For this review, take the finished solid that the model builds, in its own axes (mm). Give positions to 0.01 mm unless a question says otherwise; leave off trailing zeros. Loops run counter-clockwise (first coordinate to the right, second up) from the corner with the lowest first, then second, coordinate; pieces in that order, holes last. Notation, with made-up numbers: (30.25, 75.5) -> (87.25, 75.5) arc R18 ccw to (87.25, 95.5) -> close; hole circle Ø2 at (83.25, 81.25). An arc over 180 degrees is marked (long way). One line per question, with ' | ' between items. Start each with the question number.
(1) Consider section C-C (z = 14). Write out the cut boundary in (x, y).
(2) Consider section B-B (z = 2). Write out the cut boundary in (x, y).
(3) Wall thickness on probe 1 along Z at (x, y) = (59.5, 0.5); probe 2 along X at (y, z) = (2.85, 2.5); probe 3 along Z at (x, y) = (-61.5, 1.9): over which ranges is each line inside the solid? List them lowest first.
(4) Consider section D-D (y = 1.05). Give the number of separate pieces and of enclosed holes in the cut face, and give its area (3 significant figures).
(5) Consider section A-A (x = 59.5). Write out the cut boundary in (y, z), and give its area (3 significant figures).
(6) Insertion check: P1, Ø3.5, axis at x = 6.22, z = -8.15, coming from the -Y side; P2, Ø0.9, axis at y = 1, z = -27, coming from the +X side; P3, Ø0.9, axis at y = 2, z = -31.5, coming from the -X side. Each pin has a flat end and moves straight along its axis. Give the tip position at first contact, or say it passes through.
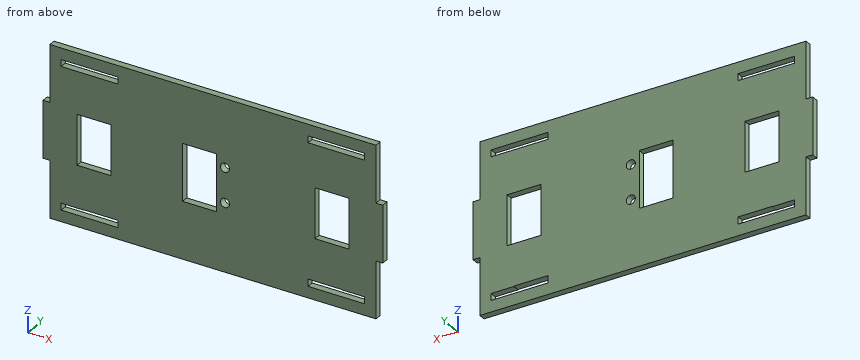
Autodesk Inventor part; units mm, degrees
ref_plane "YZ Plane" through (0, 0, 0) normal (1, 0, 0) x (0, 1, 0)
ref_plane "XZ Plane" through (0, 0, 0) normal (0, 1, 0) x (-1, 0, 0)
ref_plane "XY Plane" through (0, 0, 0) normal (0, 0, 1) x (1, 0, 0)
sketch "Sketch1" plane through (0, 0, 0) normal (0, 1, 0) x (-1, 0, 0)
  line L0 (71.1097, -38.0648) -> (71.1097, -13.0648)
  line L1 (71.1097, -13.0648) -> (74.1097, -13.0648)
  line L2 (74.1097, -13.0648) -> (74.1097, 11.9352)
  line L3 (74.1097, 11.9352) -> (71.1097, 11.9352)
  line L4 (71.1097, 11.9352) -> (71.1097, 36.9352)
  line L5 (-72.8903, -38.0648) -> (-72.8903, -13.0648)
  line L6 (-72.8903, 36.9352) -> (-72.8903, 11.9352)
  line L7 (-72.8903, -13.0648) -> (-75.8903, -13.0648)
  line L8 (-75.8903, -13.0648) -> (-75.8903, 11.9352)
  line L9 (-75.8903, 11.9352) -> (-72.8903, 11.9352)
  line L10 (71.1097, -38.0648) -> (-72.8903, -38.0648)
  line L11 (71.1097, 36.9352) -> (-72.8903, 36.9352)
  point P0 (0, 0)
extrude "Extrusion1" add sketch "Sketch1" along normal blind 3
sketch "Sketch2" plane through (0, 3, 0) normal (0, 1, 0) x (1, 0, 0)
  line L0 (-71.1097, -36.9352) -> (72.8903, -36.9352)
  line L1 (-66.1097, -31.9352) -> (-56.1097, -31.9352)
  line L2 (-56.1097, -31.9352) -> (-56.1097, -28.9352)
  line L3 (-56.1097, -28.9352) -> (-66.1097, -28.9352)
  line L4 (-66.1097, -28.9352) -> (-66.1097, -31.9352)
  line L5 (72.8903, 38.0648) -> (-71.1097, 38.0648)
  line L6 (-56.1097, 30.0648) -> (-66.1097, 30.0648)
  line L7 (-66.1097, 30.0648) -> (-66.1097, 33.0648)
  line L8 (-66.1097, 33.0648) -> (-56.1097, 33.0648)
  line L9 (-56.1097, 33.0648) -> (-56.1097, 30.0648)
  line L10 (67.8903, 33.0648) -> (57.8903, 33.0648)
  line L11 (57.8903, 33.0648) -> (57.8903, 30.0648)
  line L12 (57.8903, 30.0648) -> (67.8903, 30.0648)
  line L13 (67.8903, 30.0648) -> (67.8903, 33.0648)
  line L14 (67.8903, -31.9352) -> (57.8903, -31.9352)
  line L15 (57.8903, -31.9352) -> (57.8903, -28.9352)
  line L16 (57.8903, -28.9352) -> (67.8903, -28.9352)
  line L17 (67.8903, -28.9352) -> (67.8903, -31.9352)
  point P0 (0, 0)
extrude "Extrusion2" cut sketch "Sketch2" against normal blind 30
sketch "Sketch3" plane through (0, 3, 0) normal (0, 1, 0) x (1, 0, 0)
  line L0 (72.8903, 38.0648) -> (-71.1097, 38.0648)
  line L1 (-71.1097, -36.9352) -> (72.8903, -36.9352)
  line L2 (-74.1097, 13.0648) -> (-74.1097, -11.9352)
  line L3 (75.8903, -11.9352) -> (75.8903, 13.0648)
  circle A0 centre (6.2215, -7.0252) radius 2
  circle A1 centre (6.2215, 8.1548) radius 2
  line L4 (2.4888, 13.0648) -> (-12.5112, 13.0648)
  line L5 (-12.5112, 13.0648) -> (-12.5112, -11.9352)
  line L6 (-12.5112, -11.9352) -> (2.4888, -11.9352)
  line L7 (2.4888, -11.9352) -> (2.4888, 13.0648)
  line L8 (-59.1097, -10.4352) -> (-44.1097, -10.4352)
  line L9 (-44.1097, -10.4352) -> (-44.1097, 11.5648)
  line L10 (-44.1097, 11.5648) -> (-59.1097, 11.5648)
  line L11 (-59.1097, 11.5648) -> (-59.1097, -10.4352)
  line L12 (60.8903, 11.5648) -> (45.8903, 11.5648)
  line L13 (45.8903, 11.5648) -> (45.8903, -10.4352)
  line L14 (45.8903, -10.4352) -> (60.8903, -10.4352)
  line L15 (60.8903, -10.4352) -> (60.8903, 11.5648)
  point P0 (0, 0)
  dimension "d56" = 15
  dimension "d57" = 22
  dimension "d59" = 25
  dimension "d60" = 15
  dimension "d61" = 4
  dimension "d62" = 4
  dimension "d63" = 15
  dimension "d64" = 22
extrude "Extrusion3" cut sketch "Sketch3" against normal blind 10
sketch "Sketch4" plane through (0, 3, 0) normal (0, 1, 0) x (1, 0, 0)
  line L0 (-56.1097, 33.0648) -> (-41.1097, 33.0648)
  line L1 (-41.1097, 33.0648) -> (-41.1097, 29.924)
  line L2 (-41.1097, 29.924) -> (-56.1097, 29.924)
  line L3 (-56.1097, 29.924) -> (-56.1097, 33.0648)
  line L4 (57.8903, 30.0648) -> (57.8903, 33.0648)
  line L5 (57.8903, 33.0648) -> (42.8903, 33.0648)
  line L6 (42.8903, 33.0648) -> (42.8903, 29.924)
  line L7 (42.8903, 29.924) -> (57.8903, 29.924)
  line L8 (57.8903, 29.924) -> (57.8903, 33.0648)
  line L9 (-56.1097, -31.9352) -> (-41.1097, -31.9352)
  line L10 (-41.1097, -31.9352) -> (-41.1097, -28.9352)
  line L11 (-41.1097, -28.9352) -> (-56.1097, -28.9352)
  line L12 (-56.1097, -28.9352) -> (-56.1097, -31.9352)
  line L13 (57.8903, -31.9352) -> (57.8903, -28.9352)
  line L14 (57.8903, -28.9352) -> (42.8903, -28.9352)
  line L15 (42.8903, -28.9352) -> (42.8903, -31.9352)
  line L16 (42.8903, -31.9352) -> (57.8903, -31.9352)
  line L17 (57.8903, -31.9352) -> (57.8903, -28.9352)
  point P0 (0, 0)
  dimension "d67" = 15
  dimension "d68" = 15
extrude "Extrusion4" cut sketch "Sketch4" against normal blind 10
properties part number "Level4 (Sensor + Schakelaar)"
A:
1) outline: (-71.11, 0) -> (72.89, 0) -> (72.89, 3) -> (-71.11, 3) -> close
2) outline: (-74.11, 0) -> (-59.11, 0) -> (-59.11, 3) -> (-74.11, 3) -> close; (-44.11, 0) -> (-12.51, 0) -> (-12.51, 3) -> (-44.11, 3) -> close; (2.49, 0) -> (45.89, 0) -> (45.89, 3) -> (2.49, 3) -> close; (60.89, 0) -> (75.89, 0) -> (75.89, 3) -> (60.89, 3) -> close
3) probe 1: z = -38.06 to -33.06, -30.06 to -11.56, 10.44 to 28.94, 31.94 to 36.94 | probe 2: x = -74.11 to -59.11, -44.11 to -12.51, 2.49 to 45.89, 60.89 to 75.89 | probe 3: z = -38.06 to -33.06, -30.06 to 28.94, 31.94 to 36.94
4) separate pieces: 1 | enclosed holes: 9 | area: 9,590 mm^2
5) outline: (0, -38.06) -> (3, -38.06) -> (3, -33.06) -> (0, -33.06) -> close; (0, -30.06) -> (3, -30.06) -> (3, -11.56) -> (0, -11.56) -> close; (0, 10.44) -> (3, 10.44) -> (3, 28.94) -> (0, 28.94) -> close; (0, 31.94) -> (3, 31.94) -> (3, 36.94) -> (0, 36.94) -> close | area: 141 mm^2
6) P1: passes through | P2: stops at x = 72.89 | P3: stops at x = -71.11
